Read the model definition and answer for the solid it produces. Units are mm, in the model's axes. Face numbers are marked on the shaded views. A direction names the side the tool comes from. Give positions to 0.01 mm unless a question says otherwise; leave off trailing zeros. Order: outer loops, then holes, each group sorted by start corner. A loop starts at its lowest first (then second) coordinate and runs counter-clockwise, first axis right, second up. Notation, with made-up numbers: (83, 43.25) -> (99, 43.25) arc R12 ccw to (99, 47.25) -> close; hole circle Ø6 at (36.5, 75). An arc over 180 degrees is marked (long way). Use one line per item in the form item = value.
Solid Edge part; units mm, degrees
sketch "Sketch1" plane through (0, 0, 0) normal (0, -1, 0) x (1, 0, 0)
  line L0 (-33, -12.5) -> (33, -12.5)
  line L1 (33, -12.5) -> (33, 12.5)
  line L2 (33, 12.5) -> (-33, 12.5)
  line L3 (-33, 12.5) -> (-33, -12.5)
  dimension "D1" = 33
  dimension "D2" = 33
extrude "Protrusion1" add sketch "Sketch1" against normal blind 12
sketch "Sketch2" plane through (0, 6, -12.5) normal (0, 0, -1) x (1, 0, 0)
  line L0 (-23, 6) -> (-23, -6)
  line L1 (-23, -6) -> (-13, -6)
  line L2 (-13, 6) -> (-13, -6)
  line L3 (-23, 6) -> (-13, 6)
  line L4 (13, 6) -> (13, -6)
  line L5 (13, -6) -> (23, -6)
  line L6 (23, 6) -> (23, -6)
  line L7 (13, 6) -> (23, 6)
extrude "Extrusionsausschnitt_1" cut sketch "Sketch2" against normal blind 20
sketch "Sketch3" plane through (-33, 6, 0) normal (-1, 0, 0) x (0, -1, 0)
  line L0 (-6, 12.5) -> (6, 12.5)
  line L1 (6, 12.5) -> (6, -2.5)
  line L2 (6, -2.5) -> (-6, -2.5)
  line L3 (-6, -2.5) -> (-6, 12.5)
extrude "Extrusionsausprägung_2" add sketch "Sketch3" along normal blind 20
mirror "Mirror1" about plane through (0, 0, 0) normal (1, 0, 0) of "Extrusionsausprägung_2"
sketch "Sketch4" plane through (-33, 6, -3) normal (-1, 0, 0) x (0, -1, 0)
  circle A0 centre (-2, -2) radius 2
extrude "Extrusionsausschnitt_2" cut sketch "Sketch4" against normal blind 113.0381
sketch "Sketch5" plane through (0, 0, 0) normal (0, -1, 0) x (1, 0, 0)
  line L0 (-33, -10.5) -> (33, -10.5)
extrude "Extrusionsausschnitt_3" cut sketch "Sketch5" against normal blind 62.4108 material side at (0, 0, -10.55)
sketch "Sketch6" plane through (0, 0, 1) normal (0, -1, 0) x (1, 0, 0)
  line L0 (-53, 1.5) -> (-33, 1.5)
  line L1 (-33, 1.5) -> (-23, 11.5)
  dimension "D1" = 53
extrude "Extrusionsausschnitt_4" cut sketch "Sketch6" against normal blind 64.7066 material side at (-43, 0, 2.55)
hole "Bohrung_1" at (-48, 6, 2.5) direction (0, 0, -1) diameter 5.8 end up to next
hole "Hole1" at (-38, 6, 2.5) direction (0, 0, -1) diameter 5.8 end up to next
fillet "Verrundung_1" radius 0.5 2 edges at (-33, 6, 2.5) (-23, 6, 12.5)
chamfer "Fase_1" distance 1 angle 45 4 edges at (-23, 6, 7.5) (-13, 6, 7.5) (13, 6, 7.5) (23, 6, 7.5)
mirror "Mirror2" about plane through (0, 0, 0) normal (1, 0, 0) of "Extrusionsausschnitt_4", "Bohrung_1", "Hole1"
fillet "Round1" radius 0.5 2 edges at (33, 6, 2.5) (23, 6, 12.5)
chamfer "Chamfer1" [suppressed]
properties material "Aluminiumlegierung:3.0205, Al 99.0, EN-AW 1200"
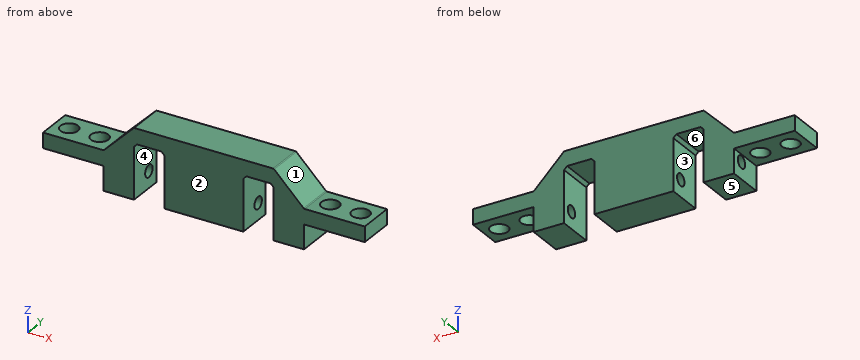
Item 1: The part is cut by section A-A on z = 0.5. Give the vertices of the cut face in (x, y).
Checks:
outline = (-53, 0) -> (-23, 0) -> (-23, 12) -> (-53, 12) -> close; (-13, 0) -> (13, 0) -> (13, 12) -> (-13, 12) -> close; (23, 0) -> (53, 0) -> (53, 12) -> (23, 12) -> close; hole circle Ø5.8 at (-48, 6); hole circle Ø5.8 at (-38, 6); hole circle Ø5.8 at (38, 6); hole circle Ø5.8 at (48, 6)
Item 2: The part is cut by section B-B on x = 36. Give the vertices of the cut face in (y, z).
Checks:
outline = (0, -2.5) -> (3.9, -2.5) -> (3.9, 2.5) -> (0, 2.5) -> close; (8.1, -2.5) -> (12, -2.5) -> (12, 2.5) -> (8.1, 2.5) -> close
Item 3: Which of the six approach directions +Z, -Z, +X, -X, +Y, -Y give full straight-line access (tool end or side, diameter ignored) to the marked faces 5 and 6?
Checks:
face_5 = -Z, +X, -X, +Y, -Y
face_6 = -Z, +Y, -Y
Item 4: Determine the mould class of the marked faces 1, 2, 3 and 4 for opening direction X: +X half, -X half, draft (parallel to the pull), parting line (faces both ways), or undercut.
Checks:
face_1 = +X half
face_2 = draft
face_3 = undercut
face_4 = undercut
Item 5: Straight lines are drawn through the part: L1, parallel to X at y = 3, z = -9.5; L2, parallel to Y at x = 38, z = -1.15; L3, parallel to Z at x = 28, y = 8. For each, find the intervals that lie inside material, in ascending order. Write a range as from..to.
Checks:
L1 = -33..-23, -13..13, 23..33
L2 = 0..3.1, 8.9..12
L3 = -10.5..-7, -3..7.5
Item 6: Given pin 1 Ø3.5 at (x, y) = (-44.5, 8.5) entering from +Z; pin 2 Ø12 at (x, z) = (38, 9.5) entering from +Y; pin 3 Ø6.5 at (y, z) = (8, -5) entering from +X; pin 4 Ø5 at (y, z) = (7, 7.5) entering from +X, each flat-ended and moving along its own axis, determine where each tip first touches the part or whether it passes through.
Checks:
pin_1 = 2.5
pin_2 = through
pin_3 = 53
pin_4 = 30.5
Item 7: The part is cut by section C-C on y = 11. Give the vertices of the cut face in (x, z), and give its area (3 significant figures).
Checks:
outline = (-53, -2.5) -> (-33, -2.5) -> (-33, -10.5) -> (-23, -10.5) -> (-23, 6.5) -> (-22, 7.5) -> (-14, 7.5) -> (-13, 6.5) -> (-13, -10.5) -> (13, -10.5) -> (13, 6.5) -> (14, 7.5) -> (22, 7.5) -> (23, 6.5) -> (23, -10.5) -> (33, -10.5) -> (33, -2.5) -> (53, -2.5) -> (53, 2.5) -> (33.21, 2.5) arc R0.5 cw to (32.85, 2.65) -> (23.15, 12.35) arc R0.5 ccw to (22.79, 12.5) -> (-22.79, 12.5) arc R0.5 ccw to (-23.15, 12.35) -> (-32.85, 2.65) arc R0.5 cw to (-33.21, 2.5) -> (-53, 2.5) -> close
area = 1,260 mm²
Item 8: The part is cut by section D-D on z = -6. Give the vertices of the cut face in (x, y), and give its area (3 significant figures).
Checks:
outline = (-33, 0) -> (-23, 0) -> (-23, 6.27) -> (-33, 6.27) -> close; (-33, 9.73) -> (-23, 9.73) -> (-23, 12) -> (-33, 12) -> close; (-13, 0) -> (13, 0) -> (13, 6.27) -> (-13, 6.27) -> close; (-13, 9.73) -> (13, 9.73) -> (13, 12) -> (-13, 12) -> close; (23, 0) -> (33, 0) -> (33, 6.27) -> (23, 6.27) -> close; (23, 9.73) -> (33, 9.73) -> (33, 12) -> (23, 12) -> close
area = 393 mm²
